```python
from build123d import *

# Parameters (mm, degrees)
SKETCH1_W           = 50
SKETCH1_H           = 23
BOSS_EXTRUDE1_DEPTH = 1
SKETCH2_R           = 0.5
CUT_EXTRUDE1_DEPTH  = 2


with BuildPart() as part:
    # Sketch1 → Boss-Extrude1 (new body)
    with BuildSketch(Plane(origin=(0, 0, 0), x_dir=(1, 0, 0), z_dir=(0, 1, 0))):
        with Locations((25, 11.5)):
            Rectangle(SKETCH1_W, SKETCH1_H)
    extrude(amount=BOSS_EXTRUDE1_DEPTH)

    # Sketch2 → Cut-Extrude1 (cut, through all)
    with BuildSketch(Plane(origin=(0, 1, 0), x_dir=(1, 0, 0), z_dir=(0, 1, 0))):
        with Locations((1.66, 3.83)):
            Circle(SKETCH2_R)
        with Locations((4.2, 3.83)):
            Circle(SKETCH2_R)
        with Locations((1.66, 6.37)):
            Circle(SKETCH2_R)
        with Locations((1.66, 8.91)):
            Circle(SKETCH2_R)
        with Locations((1.66, 11.45)):
            Circle(SKETCH2_R)
        with Locations((1.66, 13.99)):
            Circle(SKETCH2_R)
        with Locations((1.66, 16.53)):
            Circle(SKETCH2_R)
        with Locations((1.66, 19.07)):
            Circle(SKETCH2_R)
        with Locations((4.2, 6.37)):
            Circle(SKETCH2_R)
        with Locations((4.2, 8.91)):
            Circle(SKETCH2_R)
        with Locations((4.2, 11.45)):
            Circle(SKETCH2_R)
        with Locations((4.2, 13.99)):
            Circle(SKETCH2_R)
        with Locations((4.2, 16.53)):
            Circle(SKETCH2_R)
        with Locations((4.2, 1.29)):
            Circle(SKETCH2_R)
        with Locations((9.28, 19.07)):
            Circle(SKETCH2_R)
        with Locations((11.82, 19.07)):
            Circle(SKETCH2_R)
        with Locations((14.36, 19.07)):
            Circle(SKETCH2_R)
        with Locations((11.82, 21.61)):
            Circle(SKETCH2_R)
        with Locations((19.44, 21.61)):
            Circle(SKETCH2_R)
        with Locations((21.98, 21.61)):
            Circle(SKETCH2_R)
        with Locations((24.52, 21.61)):
            Circle(SKETCH2_R)
        with Locations((27.06, 21.61)):
            Circle(SKETCH2_R)
        with Locations((32.14, 21.61)):
            Circle(SKETCH2_R)
        with Locations((34.68, 21.61)):
            Circle(SKETCH2_R)
        with Locations((37.22, 21.61)):
            Circle(SKETCH2_R)
        with Locations((42.3, 21.61)):
            Circle(SKETCH2_R)
        with Locations((47.38, 21.61)):
            Circle(SKETCH2_R)
        with Locations((24.52, 1.29)):
            Circle(SKETCH2_R)
        with Locations((27.06, 1.29)):
            Circle(SKETCH2_R)
        with Locations((29.6, 1.29)):
            Circle(SKETCH2_R)
        with Locations((32.14, 1.29)):
            Circle(SKETCH2_R)
        with Locations((37.22, 1.29)):
            Circle(SKETCH2_R)
    extrude(amount=-CUT_EXTRUDE1_DEPTH, mode=Mode.SUBTRACT)


solid = part.part
```
Input: part model. Units: mm. Frame: model coordinates. Coordinates: 2 decimals unless noted, no trailing zeros. Write each loop counter-clockwise with the first axis right and the second up, starting at its lowest first coordinate (ties: lowest second). Pieces come first, ordered by that corner, then holes. Notation, with made-up numbers: M -13.5,88.5 L 37.5,88.5 A20 cw 37.5,103.5 Z; hole C -9,37 d11. An arc over 180 degrees is marked long. Use one line per item in the form item = value.
Q1. Material intervals for probe 1 along Z at (x, y) = (27.06, 0.65); probe 2 along Z at (x, y) = (11.82, 0.25); probe 3 along X at (y, z) = (0.25, -11.25), sorted ascending. Write a range as from..to.
Answer below:
probe_1 = -23..-22.11, -21.11..-1.79, -0.79..0
probe_2 = -23..-22.11, -21.11..-19.57, -18.57..0
probe_3 = 0..1.2, 2.12..3.74, 4.66..50
Q2. Section A-A (x = 4.2). Count the separate pieces of the cut face and the enclosed holes in it, plus the area to 3 significant figures.
Answer below:
separate_pieces = 8
enclosed_holes = 0
area = 16.0 mm²
Q3. Section C-C (x = 14.36). Return loops of the section in (y, z).
Answer below:
outline = M 0,-23 L 1,-23 L 1,-19.57 L 0,-19.57 Z; M 0,-18.57 L 1,-18.57 L 1,0 L 0,0 Z
Q4. Section B-B (z = -3.83). Return loops of the section in (x, y).
Answer below:
outline = M 0,0 L 1.16,0 L 1.16,1 L 0,1 Z; M 2.16,0 L 3.7,0 L 3.7,1 L 2.16,1 Z; M 4.7,0 L 50,0 L 50,1 L 4.7,1 Z
Q5. Draft query along Z for faces 1 (the face through (24.7, 0.5, -23)), 2 (the face through (47.842, 0.507, -21.418)), 3 (the face through (0, 0.5, -11.3)). Return one class per face: released by +Z, released by -Z, zero draft, split by the parting line, or undercut.
Answer below:
face_1 = released by -Z
face_2 = undercut
face_3 = zero draft
